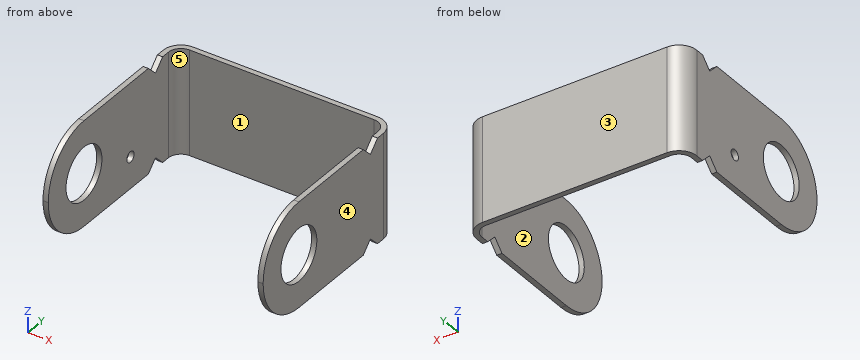
from build123d import *

# Parameters (mm, degrees)
BASE_FLANGE1_DEPTH          = 50
CUT_EXTRUDE1_DEPTH          = 285.297379517
CUT_EXTRUDE1_DEPTH_BACK     = 285.297379517
M12X1_75_TAPPED_HOLE1_D     = 10.2
M12X1_75_TAPPED_HOLE1_DEPTH = 5
BREAK_CORNER2_START         = -105
BREAK_CORNER2_DEPTH         = 210
CUT_EXTRUDE2_DEPTH          = 285.297379517
CUT_EXTRUDE2_DEPTH_BACK     = 285.297379517
SKETCH10_R                  = 25.1


# Read off the part's stored shape, not the designer's step: Break-Corner2
# Sheet-metal steps are written as plain solids
with BuildPart() as part:
    # Sketch1 → Base-Flange1 (new, symmetric)
    with BuildSketch(Plane.XY):
        with BuildLine():
            Line((-105, 0), (-105, 168))
            ThreePointArc((-105, 168), (-100.02081528, 180.02081528), (-88, 185))
            Line((-88, 185), (88, 185))
            ThreePointArc((88, 185), (100.02081528, 180.02081528), (105, 168))
            Line((105, 168), (105, 0))
            Line((105, 0), (100, 0))
            Line((100, 0), (100, 168))
            ThreePointArc((100, 168), (96.485281374, 176.485281374), (88, 180))
            Line((88, 180), (-88, 180))
            ThreePointArc((-88, 180), (-96.485281374, 176.485281374), (-100, 168))
            Line((-100, 168), (-100, 0))
            Line((-100, 0), (-105, 0))
        make_face()
    extrude(amount=BASE_FLANGE1_DEPTH, both=True)

    # Sketch6 → Cut-Extrude1 (cut, two sides: drawn at the far end of the back side and taken through both)
    with BuildSketch(Plane.ZY.offset(105).offset(-CUT_EXTRUDE1_DEPTH_BACK)):
        Polygon((-50, 160), (-40, 150), (-50, 140), align=None)
        Polygon((50, 160), (50, 140), (40, 150), align=None)
    extrude(amount=CUT_EXTRUDE1_DEPTH + CUT_EXTRUDE1_DEPTH_BACK, mode=Mode.SUBTRACT)

    # M12x1.75 Tapped Hole1
    with Locations(Plane.ZY.offset(105)):
        with Locations((-20, 115)):
            Hole(M12X1_75_TAPPED_HOLE1_D / 2, depth=M12X1_75_TAPPED_HOLE1_DEPTH)

    # Break-Corner2 outline → Break-Corner2 (cut)
    with BuildSketch(Plane.YZ.offset(BREAK_CORNER2_START)):
        with BuildLine():
            Line((0, -50), (50, -50))
            ThreePointArc((50, -50), (14.644660941, -35.355339059), (0, 0))
            Line((0, 0), (0, -50))
        make_face()
        with BuildLine():
            Line((0, 50), (0, 0))
            ThreePointArc((0, 0), (14.644660941, 35.355339059), (50, 50))
            Line((50, 50), (0, 50))
        make_face()
    extrude(amount=BREAK_CORNER2_DEPTH, mode=Mode.SUBTRACT)

    # Sketch10 → Cut-Extrude2 (cut, two sides: drawn at the far end of the back side and taken through both)
    with BuildSketch(Plane.ZY.offset(105).offset(-CUT_EXTRUDE2_DEPTH_BACK)):
        with Locations(Location((0, 50, 0), (0, 0, 270))):
            Circle(SKETCH10_R)
    extrude(amount=CUT_EXTRUDE2_DEPTH + CUT_EXTRUDE2_DEPTH_BACK, mode=Mode.SUBTRACT)


solid = part.part
Verification items for the finished model (mm, model axes). Face numbers are marked on the shaded views. A direction names the side the tool comes from. Round coordinates to 2 decimals unless told otherwise and drop trailing zeros. Loops run counter-clockwise (first coordinate to the right, second up) from the corner with the lowest first, then second, coordinate; pieces in that order, holes last. Notation, with made-up numbers: (45.5, -36) - (60.5, -36) arc R28 ccw to (60.5, -7) - close; hole circle Ø7 at (70.25, 37.5). An arc over 180 degrees is marked (long way). Use a Markdown table: item, result. Add a question column.
1. Release check for a two-part mould opening along Y. For the marked faces 1, 2 and 3 record: released by +Y, released by -Y, zero draft, split by the parting line, or undercut.
2. Gauge pin test, flat end, axial feed: pin 1 (1.5 mm diameter, centred on x = -81.5, z = -38, fed in from -Y). Record the tip position at first contact, or that the pin passes through.
3. Section check A-A, the plane y = 157. Record the boundary of the cut face in (x, z).
4. Section check D-D, the plane z = -20. Record the boundary of the cut face in (x, y).
5. Section check B-B, the plane y = 115. Record the boundary of the cut face in (x, z), plus the area to 3 significant figures.
6. Thickness scan on probe 1 along Z at (x, y) = (102, 50); probe 2 along X at (y, z) = (126, 40); probe 3 along Y at (x, z) = (72, -36). Record the ranges inside material, lowest first. Write a range as [from, to].
7. Section check C-C, the plane z = 14. Record the boundary of the cut face in (x, y), plus the area to 3 significant figures.
8. Access from +Z, -Z, +X, -X, +Y, -Y to the whole of each face (thin tool, end or side, straight path). Record for the marked faces 4 and 5.
Checks:
| question | item | result |
|---|---|---|
| 1 | face 1 | released by -Y |
| 1 | face 2 | zero draft |
| 1 | face 3 | released by +Y |
| 2 | pin 1 | stops at y = 180 |
| 3 | outline | (-105, -47) - (-100, -47) - (-100, 47) - (-105, 47) - close; (100, -47) - (105, -47) - (105, 47) - (100, 47) - close |
| 4 | outline | (-105, 4.17) - (-100, 4.17) - (-100, 34.83) - (-105, 34.83) - close; (-105, 65.17) - (-100, 65.17) - (-100, 109.9) - (-105, 109.9) - close; (-105, 120.1) - (-100, 120.1) - (-100, 168) arc R12 cw to (-88, 180) - (88, 180) arc R12 cw to (100, 168) - (100, 65.17) - (105, 65.17) - (105, 168) arc R17 ccw to (88, 185) - (-88, 185) arc R17 ccw to (-105, 168) - close; (100, 4.17) - (105, 4.17) - (105, 34.83) - (100, 34.83) - close |
| 5 | outline | (-105, -50) - (-100, -50) - (-100, -25.1) - (-105, -25.1) - close; (-105, -14.9) - (-100, -14.9) - (-100, 50) - (-105, 50) - close; (100, -50) - (105, -50) - (105, 50) - (100, 50) - close |
| 5 | area | 949 mm^2 |
| 6 | probe 1 | z = [-50, -25.1], [25.1, 50] |
| 6 | probe 2 | x = [-105, -100], [100, 105] |
| 6 | probe 3 | y = [180, 185] |
| 7 | outline | (-105, 2) - (-100, 2) - (-100, 29.17) - (-105, 29.17) - close; (-105, 70.83) - (-100, 70.83) - (-100, 168) arc R12 cw to (-88, 180) - (88, 180) arc R12 cw to (100, 168) - (100, 70.83) - (105, 70.83) - (105, 168) arc R17 ccw to (88, 185) - (-88, 185) arc R17 ccw to (-105, 168) - close; (100, 2) - (105, 2) - (105, 29.17) - (100, 29.17) - close |
| 7 | area | 2,350 mm^2 |
| 8 | face 4 | +Z, -Z, +X, +Y, -Y |
| 8 | face 5 | +Z, -Z, -Y |
